Check sheet for the modelled part. Datum: model origin and axes. Units: mm. Face numbers are marked on the shaded views. A direction names the side the tool comes from. Coordinates: 2 decimals unless noted, no trailing zeros. Order: outer loops, then holes, each group sorted by start corner. A loop starts at its lowest first (then second) coordinate and runs counter-clockwise, first axis right, second up.
1. Cross-section at B-B (x = 45). Enter the section's corners in (y, z).
2. Draft check along X on the marked faces 1, 2 and 3. Enter one of: released by +X, released by -X, zero draft, split by the parting line, or undercut.
3. Gauge pin test, flat ends, axial feed: pin 1 Ø4 at (x, z) = (42, 12.5) entering from -Y; pin 2 Ø1.8 at (x, z) = (25, 12.5) entering from -Y. Record the tip position at first contact, or that the pin passes through.
4. Thickness scan on line 1 (Z direction, x = 42, y = -29.15); line 2 (Y direction, x = 32, z = 4.5); line 3 (X direction, y = -9.75, z = 16.25). Record the ranges inside material, lowest first.
5. Cross-section at C-C (y = -6.25). Enter the section's corners in (x, z).
6. Cross-section at D-D (x = 8). Enter the section's corners in (y, z).
7. Set-up check for the marked faces 4 and 5: record each of +Z, -Z, +X, -X, +Y, -Y from which the full face is reachable in a straight line by a thin tool's end or side.
8. Cross-section at A-A (z = 12.5). Count the separate pieces of the cut face and the enclosed holes in it, then the cut area to 3 significant figures.
```python
from build123d import *

# Parameters (mm, degrees)
F0_W     = 50
F0_H     = 30
F0_W_2   = 42
F0_H_2   = 22
F1_DEPTH = 25
F2_R     = 1.5
F3_DEPTH = 35


with BuildPart() as f1:
    # F0 (on Top) → F1 (new body)
    with BuildSketch(Plane.XY):
        with Locations((25, -15)):
            Rectangle(F0_W, F0_H)
        with Locations((25, -15)):
            Rectangle(F0_W_2, F0_H_2, mode=Mode.SUBTRACT)
    extrude(amount=F1_DEPTH)

    # F2 (on face) → F3 (cut)
    with BuildSketch(Plane.XZ.offset(30)):
        with Locations((25, 12.5)):
            Circle(F2_R)
        with Locations((8, 12.5)):
            Circle(F2_R)
        with Locations((42, 12.5)):
            Circle(F2_R)
    extrude(amount=-F3_DEPTH, mode=Mode.SUBTRACT)


solid = f1.part
```
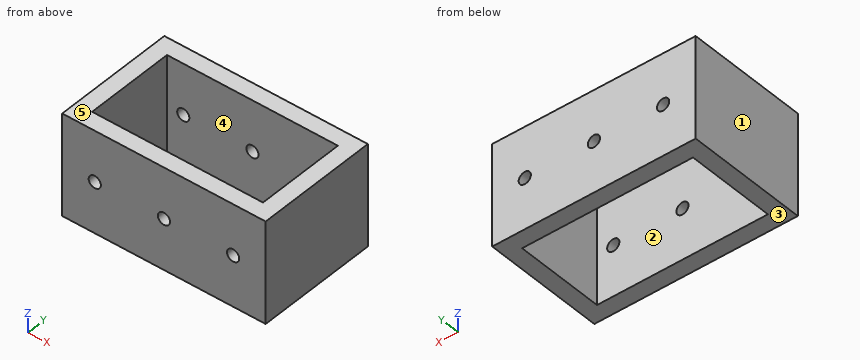
Data:
1. outline: (-30, 0) - (-26, 0) - (-26, 25) - (-30, 25) - close; (-4, 0) - (0, 0) - (0, 25) - (-4, 25) - close
2. face 1: released by -X
2. face 2: undercut
2. face 3: zero draft
3. pin 1: stops at y = -30
3. pin 2: passes through
4. line 1: z = 0 to 11, 14 to 25
4. line 2: y = -30 to -26, -4 to 0
4. line 3: x = 0 to 4, 46 to 50
5. outline: (0, 0) - (4, 0) - (4, 25) - (0, 25) - close; (46, 0) - (50, 0) - (50, 25) - (46, 25) - close
6. outline: (-30, 0) - (-26, 0) - (-26, 11) - (-30, 11) - close; (-30, 14) - (-26, 14) - (-26, 25) - (-30, 25) - close; (-4, 0) - (0, 0) - (0, 11) - (-4, 11) - close; (-4, 14) - (0, 14) - (0, 25) - (-4, 25) - close
7. face 4: +Z, -Z
7. face 5: +Z, +X, -X, +Y, -Y
8. separate pieces: 6
8. enclosed holes: 0
8. area: 504 mm2
